Here's the drawing with two shaded views (mm, measured from the low corner). I have some questions. A direction names the side the tool comes from. Round coordinates to 2 decimals unless told otherwise and drop trailing zeros. Loops run counter-clockwise (first coordinate to the right, second up) from the corner with the lowest first, then second, coordinate; pieces in that order, holes last. Notation, with made-up numbers: (52, -34.5) -> (68, -34.5) arc R26 cw to (68, -19.5) -> close; hole circle Ø11 at (-18.5, 29). An arc over 180 degrees is marked (long way). Write item = value, one per line.
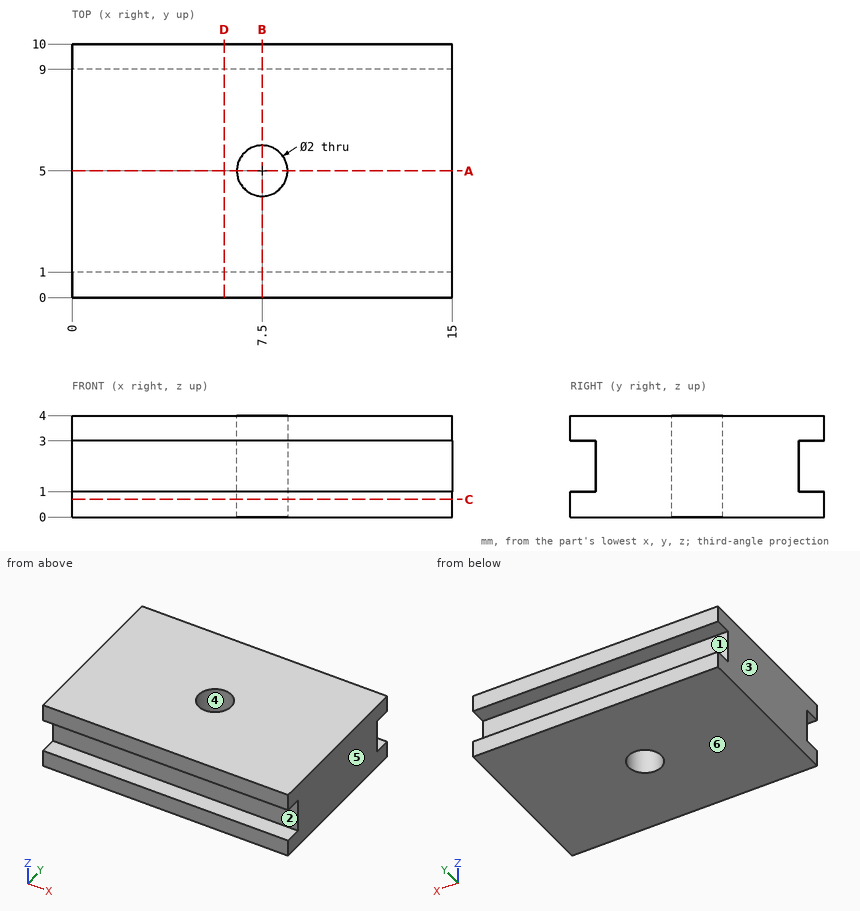
1. Suppose I cut it at C-C, the plane z = 0.7. List the corners of the cut face in (x, y) for me, and give its area (3 significant figures).
Entries:
outline = (0, 0) -> (15, 0) -> (15, 10) -> (0, 10) -> close; hole circle Ø2 at (7.5, 5)
area = 147 mm²
2. Suppose I cut it at B-B, the plane x = 7.5. List the corners of the cut face in (y, z) for me, and give its area (3 significant figures).
Entries:
outline = (0, 0) -> (4, 0) -> (4, 4) -> (0, 4) -> (0, 3) -> (1, 3) -> (1, 1) -> (0, 1) -> close; (6, 0) -> (10, 0) -> (10, 1) -> (9, 1) -> (9, 3) -> (10, 3) -> (10, 4) -> (6, 4) -> close
area = 28.0 mm²
3. I need wall thicknesses on line 1 (Z direction, x = 6, y = 0.5); line 2 (Y direction, x = 7.5, z = 0.8); line 3 (X direction, y = 5.25, z = 0.8). Which ranges of each line are inside material? Lowest first, please. Write a range as [from, to].
Entries:
line_1 = [0, 1], [3, 4]
line_2 = [0, 4], [6, 10]
line_3 = [0, 6.53], [8.47, 15]
4. Suppose I cut it at D-D, the plane x = 6. List the corners of the cut face in (y, z) for me, and give its area (3 significant figures).
Entries:
outline = (0, 0) -> (10, 0) -> (10, 1) -> (9, 1) -> (9, 3) -> (10, 3) -> (10, 4) -> (0, 4) -> (0, 3) -> (1, 3) -> (1, 1) -> (0, 1) -> close
area = 36.0 mm²
5. For the marked faces 1, 2 and 3, which set-ups out of +Z, -Z, +X, -X, +Y, -Y let a thin tool reach every point of the face, with its end or its side?
Entries:
face_1 = +X, -X, +Y
face_2 = +X, -X, -Y
face_3 = +Z, -Z, -X, +Y, -Y
6. I'm going to push a flat-ended pin straight in: pin 1 (1.6 mm diameter, centred on x = 4.5, z = 2, fed in from +Y). Where does the tip first touch, or does it pass through?
Entries:
pin_1 = 9
7. We'd pull the mould along X, two halves only. Please class the marked faces 4, 5 and 6: released by +X, released by -X, zero draft, split by the parting line, or undercut.
Entries:
face_4 = undercut
face_5 = released by +X
face_6 = zero draft
8. Suppose I cut it at A-A, the plane y = 5. List the corners of the cut face in (x, z) for me, and give its area (3 significant figures).
Entries:
outline = (0, 0) -> (6.5, 0) -> (6.5, 4) -> (0, 4) -> close; (8.5, 0) -> (15, 0) -> (15, 4) -> (8.5, 4) -> close
area = 52.0 mm²
